Geometry: final body of the model. Coordinates: model frame, mm. Give positions to 0.01 mm unless a question says otherwise; leave off trailing zeros. Write each loop counter-clockwise with the first axis right and the second up, starting at its lowest first coordinate (ties: lowest second). Pieces come first, ordered by that corner, then holes. Notation, with made-up numbers: M 17.25,-17.75 L 76.25,-17.75 A16 ccw 76.25,11.25 Z; hole C 72.25,23 d10. An arc over 180 degrees is marked long. Use a Markdown table: item, result. Add a question column.
1) Line query: line 1 (Z direction, x = 755.5, y = 181) (3 decimals); line 2 (X direction, y = 179, z = -14); line 3 (Z direction, x = 747, y = 186) (3 decimals). Output: solid intervals per line, ascending.
2) Section A-A on x = 750.5. Return the cut outline in (y, z) (1 decimal), then the cut area to 3 significant figures.
3) Section B-B on y = 195.5. Return the cut outline in (x, z) (1 decimal).
4) Pin query (flat end, axial travel): pin 1 (10 mm diameter, centred on x = 750.5, z = -100.5, fed in from +Y). Return the tip coordinate at first contact, or that it passes through.
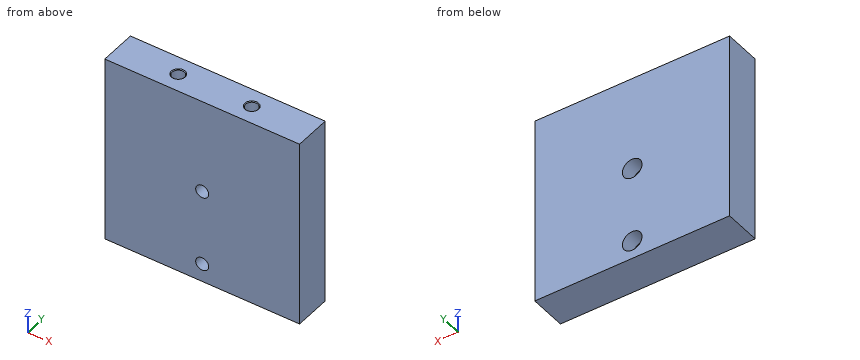
```python
from build123d import *

# Parameters (mm, degrees)
F0_W           = 201.93
F0_H           = 196.215
F0_R           = 10.16
F0_R_2         = 6.604
F1_DEPTH       = 38.1
F2_D           = 13.462
F2_DEPTH       = 50.8
F2_CBORE_D     = 20.32
F2_CBORE_DEPTH = 15.875
F2_TIP         = 4.0443928267
F3_ANGLE       = -90
F5_D           = 12.7
F5_DEPTH       = 34.925
F5_CSINK_D     = 14.2875
F5_CSINK_ANGLE = 90
F5_TIP         = 3.8154649308


with BuildPart() as f1:
    # F0 (on Top) → F1 (new body)
    with BuildSketch(Plane.XY):
        with Locations((754.8313072, 347.5162722)):
            Rectangle(F0_W, F0_H)
        with Locations((754.8313072, 268.4587722)):
            Circle(F0_R, mode=Mode.SUBTRACT)
        with Locations((754.8313072, 347.5162722)):
            Circle(F0_R, mode=Mode.SUBTRACT)
        with Locations((754.8313072, 426.5737722)):
            Circle(F0_R, mode=Mode.SUBTRACT)
        with Locations((754.8313072, 426.5737722)):
            Circle(F0_R)
        with Locations((754.8313072, 426.5737722)):
            Circle(F0_R_2, mode=Mode.SUBTRACT)
        with Locations((754.8313072, 347.5162722)):
            Circle(F0_R)
        with Locations((754.8313072, 347.5162722)):
            Circle(F0_R_2, mode=Mode.SUBTRACT)
        with Locations((754.8313072, 347.5162722)):
            Circle(F0_R_2)
        with Locations((754.8313072, 426.5737722)):
            Circle(F0_R_2)
        with Locations((754.8313072, 268.4587722)):
            Circle(F0_R)
        with Locations((754.8313072, 268.4587722)):
            Circle(F0_R_2, mode=Mode.SUBTRACT)
        with Locations((754.8313072, 268.4587722)):
            Circle(F0_R_2)
    extrude(amount=-F1_DEPTH)

    # F2
    with Locations(Plane.XY):
        with Locations((754.8313072, 426.5737722), (754.8313072, 347.5162722)):
            CounterBoreHole(F2_D / 2, F2_CBORE_D / 2, F2_CBORE_DEPTH, depth=F2_DEPTH)
            with Locations((0, 0, -(F2_DEPTH + F2_TIP / 2))):  # 118° drill point
                Cone(0, F2_D / 2, F2_TIP, mode=Mode.SUBTRACT)


with BuildPart() as f1_1:
    # F3: moved
    add(f1.part.rotate(Axis((754.8313072, 249.4087722, 0), (1, 0, 0)), F3_ANGLE))


with BuildPart() as f1_2:
    # F4: moved
    add(f1_1.part.moved(Location((0, -50.8, 0))))

    # F5
    with Locations(Plane.XY):
        with Locations((716.7313072, 179.5587722), (792.9313072, 179.5587722)):
            CounterSinkHole(F5_D / 2, F5_CSINK_D / 2, depth=F5_DEPTH, counter_sink_angle=F5_CSINK_ANGLE)
            with Locations((0, 0, -(F5_DEPTH + F5_TIP / 2))):  # 118° drill point
                Cone(0, F5_D / 2, F5_TIP, mode=Mode.SUBTRACT)


solid = f1_2.part
```
Found:
| question | item | result |
|---|---|---|
| 1 | line 1 | -196.215 to -183.863, -170.467 to -104.805, -91.41 to 0 |
| 1 | line 2 | 653.87 to 710.41, 723.06 to 786.61, 799.26 to 855.8 |
| 1 | line 3 | -196.215 to -183.638, -170.692 to -104.58, -91.635 to 0 |
| 2 | outline | M 160.5,-196.2 L 198.6,-196.2 L 198.6,-186.4 L 182.7,-186.4 L 182.7,-182.3 L 160.5,-182.3 Z; M 160.5,-172 L 182.7,-172 L 182.7,-168 L 198.6,-168 L 198.6,-107.3 L 182.7,-107.3 L 182.7,-103.3 L 160.5,-103.3 Z; M 160.5,-93 L 182.7,-93 L 182.7,-88.9 L 198.6,-88.9 L 198.6,0 L 160.5,0 Z |
| 2 | area | 6,430 mm² |
| 3 | outline | M 653.9,-196.2 L 855.8,-196.2 L 855.8,0 L 653.9,0 Z; hole C 754.8,-177.2 d20.3; hole C 754.8,-98.1 d20.3 |
| 4 | pin 1 | y = 182.73 |
